Build history of the part. All positions in model axes, mm. Face numbers are marked on the shaded views. A direction names the side the tool comes from. Give positions to 0.01 mm unless a question says otherwise; leave off trailing zeros. Write each loop counter-clockwise with the first axis right and the second up, starting at its lowest first coordinate (ties: lowest second). Pieces come first, ordered by that corner, then holes.
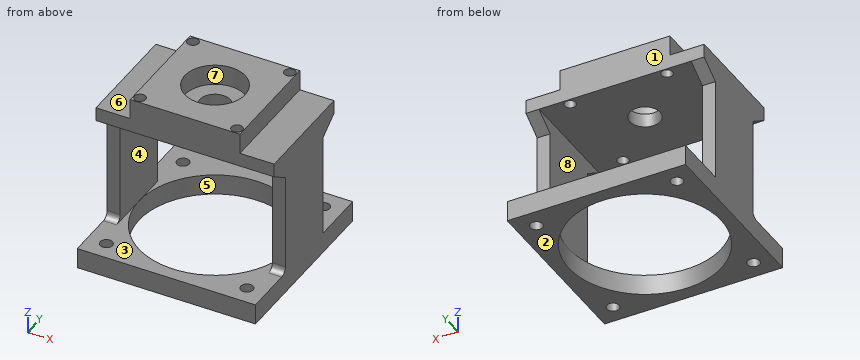
Autodesk Inventor part; units mm, degrees
ref_plane "YZ Plane" through (0, 0, 0) normal (1, 0, 0) x (0, 1, 0)
ref_plane "XZ Plane" through (0, 0, 0) normal (0, 1, 0) x (-1, 0, 0)
ref_plane "XY Plane" through (0, 0, 0) normal (0, 0, 1) x (1, 0, 0)
sketch "Sketch1" plane through (0, 0, 0) normal (0, 0, 1) x (1, 0, 0)
  line L0 (-65, 65) -> (65, 65)
  line L1 (65, 65) -> (65, -65)
  line L2 (65, -65) -> (-65, -65)
  line L3 (-65, -65) -> (-65, 65)
  line L4 (-65, 65) -> (65, -65) construction
  line L5 (65, 65) -> (-65, -65) construction
  circle A0 centre (0, 0) radius 72.5 construction
  circle A1 centre (51.2652, 51.2652) radius 4.5
  line L6 (0, 0) -> (0, 13.8436) construction
  line L7 (0, 0) -> (-14.1522, 0) construction
  circle A2 centre (-51.2652, 51.2652) radius 4.5
  circle A3 centre (51.2652, -51.2652) radius 4.5
  circle A4 centre (-51.2652, -51.2652) radius 4.5
  dimension "d66" = 145
  dimension "d0" = 130
  dimension "d1" = 130
  dimension "d67" = 9
extrude "Extrusion1" add sketch "Sketch1" along normal blind 15
sketch "Sketch2" plane through (65, -65, 0) normal (1, 0, 0) x (0, 0, -1)
  line L0 (0, 0) -> (0, 130) construction
  line L1 (-22.5, 65) -> (-82.5, 65) construction
  line L2 (-90, 40) -> (-15, 40)
  line L3 (-15, 90) -> (-15, 40)
  line L4 (-15, 0) -> (-15, 130) construction
  line L5 (-15, 90) -> (-15, 130) construction
  line L6 (-100, 105) -> (-110, 105)
  line L7 (-110, 105) -> (-110, 25)
  line L8 (-15, 90) -> (-90, 90)
  line L9 (-90, 90) -> (-100, 105)
  line L10 (-110, 25) -> (-100, 25)
  line L11 (-100, 25) -> (-90, 40)
  point P0 (0, 90)
  point P1 (0, 40)
  dimension "d98" = 10
  dimension "d101" = 110
  dimension "d102" = 75
  dimension "d103" = 75
  dimension "d104" = 10
extrude "Extrusion2" add sketch "Sketch2" against normal blind 9.5
mirror "Mirror1" about plane through (0, 0, 0) normal (1, 0, 0) of "Extrusion2"
sketch "Sketch6" plane through (0, 0, 0) normal (0, 0, -1) x (-1, 0, 0)
  circle A0 centre (0, 0) radius 55.5
  dimension "d37" = 111
extrude "Extrusion6" cut sketch "Sketch6" against normal up to surface (15 mm away)
fillet "Fillet1" radius 5 2 edges at (-60.25, -25, 15) (60.25, -25, 15)
sketch "Sketch14" plane through (-65, -40, 110) normal (0, 0, 1) x (1, 0, 0)
  line L0 (120.5, 15) -> (120.5, 0)
  line L1 (9.5, 80) -> (120.5, 80)
  line L2 (120.5, 80) -> (120.5, 0)
  line L3 (120.5, 0) -> (9.5, 0)
  line L4 (9.5, 0) -> (9.5, 80)
extrude "Extrusion14" add sketch "Sketch14" against normal blind 10
sketch "Sketch15" plane through (65, -40, 110) normal (0, 0, 1) x (1, 0, 0)
  line L0 (-25, 0) -> (-105, 0)
  line L1 (-105, 0) -> (-105, 80)
  line L2 (-105, 80) -> (-25, 80)
  line L3 (-25, 80) -> (-25, 0)
  line L4 (-25, 0) -> (-105, 80) construction
  line L5 (-105, 0) -> (-25, 80) construction
  point P0 (-65, 40)
  dimension "d105" = 80
  dimension "d106" = 80
extrude "Extrusion15" add sketch "Sketch15" along normal blind 15
sketch "Sketch16" plane through (65, -40, 125) normal (0, 0, 1) x (1, 0, 0)
  circle A0 centre (-65, 40) radius 50 construction
  line L0 (-65, 40) -> (-100.3553, 75.3553) construction
  line L1 (-65, 40) -> (-15, 40) construction
  line L2 (-65, 40) -> (-65, 52) construction
  circle A1 centre (-100.3553, 75.3553) radius 4.075
  circle A2 centre (-29.6447, 75.3553) radius 4.075
  circle A3 centre (-100.3553, 4.6447) radius 4.075
  circle A4 centre (-29.6447, 4.6447) radius 4.075
  circle A5 centre (-65, 40) radius 11.075
  dimension "d109" = 100
  dimension "d110" = 135
  dimension "d111" = 12
  dimension "d112" = 8.15
  dimension "d113" = 22.15
extrude "Extrusion16" cut sketch "Sketch16" against normal up to surface (25 mm away)
sketch "Sketch17" plane through (65, -40, 125) normal (0, 0, 1) x (1, 0, 0)
  circle A0 centre (-65, 40) radius 22.05
  circle A1 centre (-65, 40) radius 11.075
  dimension "d116" = 44.1
extrude "Extrusion17" cut sketch "Sketch17" against normal blind 15
properties part number "MOTOR-BRACKET"
1. Drill centre lines: line 1 along X through (y, z) = (-3, 58.5); line 2 along Z through (x, y) = (-45.5, 56.5); line 3 along Z through (x, y) = (-43, 14). Where is each one in solid material? Low to high.
2. Saw through at D-D on x = 49.5. Give the cut face in (y, z).
3. Drop flat-ended pins along their axis: pin 1 (11.5 mm diameter, centred on x = -51.27, y = 51.27, fed in from +Z); pin 2 (10.5 mm diameter, centred on x = 62, z = 34.5, fed in from +Y); pin 3 (22 mm diameter, centred on x = -7, y = 3, fed in from +Z); pin 4 (8 mm diameter, centred on x = 11.5, z = 93, fed in from +Y). Give the stop position or say it passes through.
4. Saw through at C-C on y = -44. Give the cut face in (x, z), plus the area to 3 significant figures.
5. Saw through at A-A on z = 70. Give the cut face in (x, y), plus the area to 3 significant figures.
6. Saw through at B-B on x = 0. Give the cut face in (y, z) (3 decimals), plus the area to 3 significant figures.
7. 3-axis set-ups, long thin cutter, end or side, ignore diameter. For the marked faces 5, 6, 7 and 8: which of +Z, -Z, +X, -X, +Y, -Y reach the whole face in a straight line?
8. Mould opens along Z. For the marked faces 1, 2, 3 and 4 say: pulls with the +Z half, pulls with the -Z half, needs draft (parallel to the pull), parting line crosses it, or undercut.
Outcome:
1. line 1: x = -65 to -55.5, 55.5 to 65
1. line 2: z = 0 to 15
1. line 3: z = 100 to 110
2. outline: (-65, 0) - (-55.4, 0) - (-55.4, 15) - (-65, 15) - close; (-47.13, 0) - (-25.1, 0) - (-25.1, 15) - (-47.13, 15) - close; (-40, 100) - (40, 100) - (40, 110) - (-40, 110) - close; (25.1, 0) - (47.13, 0) - (47.13, 15) - (25.1, 15) - close; (55.4, 0) - (65, 0) - (65, 15) - (55.4, 15) - close
3. pin 1: stops at z = 15
3. pin 2: stops at y = 25
3. pin 3: stops at z = 110
3. pin 4: passes through
4. outline: (-65, 0) - (-33.83, 0) - (-33.83, 15) - (-65, 15) - close; (33.83, 0) - (65, 0) - (65, 15) - (33.83, 15) - close
4. area: 935 mm2
5. outline: (-65, -25) - (-55.5, -25) - (-55.5, 25) - (-65, 25) - close; (55.5, -25) - (65, -25) - (65, 25) - (55.5, 25) - close
5. area: 950 mm2
6. outline: (-65, 0) - (-55.5, 0) - (-55.5, 15) - (-65, 15) - close; (-40, 100) - (-11.075, 100) - (-11.075, 110) - (-22.05, 110) - (-22.05, 125) - (-40, 125) - close; (11.075, 100) - (40, 100) - (40, 125) - (22.05, 125) - (22.05, 110) - (11.075, 110) - close; (55.5, 0) - (65, 0) - (65, 15) - (55.5, 15) - close
6. area: 1,400 mm2
7. face 5: -Z
7. face 6: +Z, -X, +Y, -Y
7. face 7: +Z
7. face 8: +Y, -Y
8. face 1: needs draft
8. face 2: pulls with the -Z half
8. face 3: undercut
8. face 4: undercut
